Could you check a few things on this model? Use its own coordinates, in mm. Coordinates: 2 decimals unless noted, no trailing zeros. Loops run counter-clockwise (first coordinate to the right, second up) from the corner with the lowest first, then second, coordinate; pieces in that order, holes last.
1) Imagine slicing it at A-A on z = -110. Please give me the cut outline in (x, y), plus the area to 3 significant figures.
2) Imagine slicing it at B-B on y = 1.15. Give the number of separate pieces and of enclosed holes in the cut face, plus the area to 3 significant figures.
3) If I drill on line 1 along X through (y, z) = (1.35, -107); line 2 along Z through (x, y) = (69, 0.6), over which ranges is the centre line in solid material (lowest first)?
```python
from build123d import *

# Parameters (mm, degrees)
SKETCH1_W               = 180
SKETCH1_H               = 270
BOSS_EXTRUDE1_DEPTH     = 3
SKETCH2_W               = 15.818181818
SKETCH2_H               = 3
SKETCH2_W_2             = 3
SKETCH2_H_2             = 17.6
CUT_EXTRUDE1_DEPTH      = 1
CUT_EXTRUDE1_DEPTH_BACK = 4
FILLET1_R               = 2.5


with BuildPart() as part:
    # Sketch1 → Boss-Extrude1 (new body)
    with BuildSketch(Plane(origin=(0, 0, 0), x_dir=(1, 0, 0), z_dir=(0, 1, 0))):
        Rectangle(SKETCH1_W, SKETCH1_H)
    extrude(amount=BOSS_EXTRUDE1_DEPTH)

    # Sketch2 → Cut-Extrude1 (cut, two sides)
    with BuildSketch(Plane(origin=(0, 3, 0), x_dir=(1, 0, 0), z_dir=(0, 1, 0))) as cut_extrude1_sk:
        with Locations((0, 130.5)):
            Rectangle(SKETCH2_W, SKETCH2_H)
        with Locations((31.636363636, 130.5)):
            Rectangle(SKETCH2_W, SKETCH2_H)
        with Locations((63.272727273, 130.5)):
            Rectangle(SKETCH2_W, SKETCH2_H)
        with Locations((85.5, -70.4)):
            Rectangle(SKETCH2_W_2, SKETCH2_H_2)
        with Locations((-31.636363636, 130.5)):
            Rectangle(SKETCH2_W, SKETCH2_H)
        with Locations((-63.272727273, 130.5)):
            Rectangle(SKETCH2_W, SKETCH2_H)
        with Locations((85.5, -105.6)):
            Rectangle(SKETCH2_W_2, SKETCH2_H_2)
        with Locations((-85.5, 105.6)):
            Rectangle(SKETCH2_W_2, SKETCH2_H_2)
        with Locations((-85.5, 70.4)):
            Rectangle(SKETCH2_W_2, SKETCH2_H_2)
        with Locations((-85.5, 35.2)):
            Rectangle(SKETCH2_W_2, SKETCH2_H_2)
        with Locations((-85.5, 0)):
            Rectangle(SKETCH2_W_2, SKETCH2_H_2)
        with Locations((85.5, 105.6)):
            Rectangle(SKETCH2_W_2, SKETCH2_H_2)
        with Locations((85.5, 70.4)):
            Rectangle(SKETCH2_W_2, SKETCH2_H_2)
        with Locations((85.5, 35.2)):
            Rectangle(SKETCH2_W_2, SKETCH2_H_2)
        with Locations((85.5, 0)):
            Rectangle(SKETCH2_W_2, SKETCH2_H_2)
        with Locations((85.5, -35.2)):
            Rectangle(SKETCH2_W_2, SKETCH2_H_2)
        with Locations((-85.5, -35.2)):
            Rectangle(SKETCH2_W_2, SKETCH2_H_2)
        with Locations((-85.5, -70.4)):
            Rectangle(SKETCH2_W_2, SKETCH2_H_2)
        with Locations((-85.5, -105.6)):
            Rectangle(SKETCH2_W_2, SKETCH2_H_2)
    extrude(amount=CUT_EXTRUDE1_DEPTH, mode=Mode.SUBTRACT)
    extrude(cut_extrude1_sk.sketch, amount=-CUT_EXTRUDE1_DEPTH_BACK, mode=Mode.SUBTRACT)

    # Fillet1
    fillet1_edges = [part.edges().sort_by_distance(p)[0] for p in [
        (90, 1.5, -135),
        (90, 1.5, 135),
        (-90, 1.5, 135),
        (-90, 1.5, -135),
    ]]
    fillet(fillet1_edges, radius=FILLET1_R)


solid = part.part
```
Filled in:
1. outline: (-90, 0) - (-87, 0) - (-87, 3) - (-90, 3) - close; (-84, 0) - (84, 0) - (84, 3) - (-84, 3) - close; (87, 0) - (90, 0) - (90, 3) - (87, 3) - close
1. area: 522 mm2
2. separate pieces: 1
2. enclosed holes: 19
2. area: 47,600 mm2
3. line 1: x = -90 to -87, -84 to 84, 87 to 90
3. line 2: z = -135 to -132, -129 to 135
